```python
from build123d import *

# Parameters (mm, degrees)
SKETCH1_R           = 2.286
BOSS_EXTRUDE1_DEPTH = 7.62
CUT_EXTRUDE1_DEPTH  = 10.16
BOSS_EXTRUDE2_DEPTH = 1.27
SKETCH4_R           = 18.415
CUT_EXTRUDE2_DEPTH  = 2.54
FILLET1_R           = 2.54


with BuildPart() as part:
    # Sketch1 → Boss-Extrude1 (new body)
    with BuildSketch(Plane(origin=(0, 0, 0), x_dir=(1, 0, 0), z_dir=(0, 1, 0))):
        Polygon((5.08, 12.7), (-5.08, 12.7), (-5.08, 10.16), (-15.24, 10.16), (-15.24, 0), (15.24, 0), (15.24, 10.16), (5.08, 10.16), align=None)
        with Locations(Location((-8.89, 5.08, 0), (0, 0, 270))):
            Circle(SKETCH1_R, mode=Mode.SUBTRACT)
        with Locations(Location((8.89, 5.08, 0), (0, 0, 90))):
            Circle(SKETCH1_R, mode=Mode.SUBTRACT)
    extrude(amount=BOSS_EXTRUDE1_DEPTH)

    # Sketch2 → Cut-Extrude1 (cut)
    with BuildSketch(Plane(origin=(5.08, 0, 0), x_dir=(0, 0, -1), z_dir=(1, 0, 0))):
        with BuildLine():
            Line((2.9845, 9.144), (15.6845, 9.144))
            ThreePointArc((15.6845, 9.144), (18.618869601, 5.27151286), (14.097, 3.494049241))
            ThreePointArc((14.097, 3.494049241), (12.5095, 3.940098483), (10.922, 3.494049241))
            ThreePointArc((10.922, 3.494049241), (9.3345, 3.048), (7.747, 3.494049241))
            ThreePointArc((7.747, 3.494049241), (6.1595, 3.940098483), (4.572, 3.494049241))
            ThreePointArc((4.572, 3.494049241), (2.9845, 3.048), (1.397, 3.494049241))
            ThreePointArc((1.397, 3.494049241), (-0.1905, 3.940098483), (-1.778, 3.494049241))
            ThreePointArc((-1.778, 3.494049241), (-2.54101286, 3.161630399), (-3.3655, 3.048))
            Line((-3.3655, 3.048), (-3.3655, 9.144))
            Line((-3.3655, 9.144), (2.9845, 9.144))
        make_face()
    extrude(amount=-CUT_EXTRUDE1_DEPTH, mode=Mode.SUBTRACT)

    # Sketch3 → Boss-Extrude2 (add, symmetric)
    with BuildSketch(Plane(origin=(0, 0, 0), x_dir=(0, 0, -1), z_dir=(1, 0, 0))):
        with BuildLine():
            Line((4.8895, 7.62), (4.8895, 6.096))
            ThreePointArc((4.8895, 6.096), (2.9845, 4.191), (1.0795, 6.096))
            Line((1.0795, 6.096), (1.0795, 7.62))
            Line((1.0795, 7.62), (0, 7.62))
            Line((0, 7.62), (0, 3.934139533))
            ThreePointArc((0, 3.934139533), (0.725327968, 3.799255708), (1.397, 3.494049241))
            ThreePointArc((1.397, 3.494049241), (2.9845, 3.048), (4.572, 3.494049241))
            ThreePointArc((4.572, 3.494049241), (6.1595, 3.940098483), (7.747, 3.494049241))
            ThreePointArc((7.747, 3.494049241), (9.3345, 3.048), (10.922, 3.494049241))
            ThreePointArc((10.922, 3.494049241), (11.777159836, 3.850811359), (12.7, 3.934139533))
            Line((12.7, 3.934139533), (12.7, 7.62))
            Line((12.7, 7.62), (11.2395, 7.62))
            Line((11.2395, 7.62), (11.2395, 6.096))
            ThreePointArc((11.2395, 6.096), (9.3345, 4.191), (7.4295, 6.096))
            Line((7.4295, 6.096), (7.4295, 7.62))
            Line((7.4295, 7.62), (4.8895, 7.62))
        make_face()
    extrude(amount=BOSS_EXTRUDE2_DEPTH, both=True)

    # Sketch4 → Cut-Extrude2 (cut, symmetric)
    with BuildSketch(Plane(origin=(0, 0, 0), x_dir=(0, 0, -1), z_dir=(1, 0, 0))):
        with Locations((21.336, -10.18977017)):
            Circle(SKETCH4_R)
    extrude(amount=CUT_EXTRUDE2_DEPTH, both=True, mode=Mode.SUBTRACT)


with BuildPart() as cut_extrude2_kept_piece:
    # of the separate pieces the step leaves, the one the design keeps (cut_extrude2_pieces_kept)
    add(part.part.solids().sort_by_distance((5.08, 0, -12.7))[0])

    # Fillet1
    fillet1_edges = [cut_extrude2_kept_piece.edges().sort_by_distance(p)[0] for p in [
        (0, 4.301003177, -9.972474456),
    ]]
    fillet(fillet1_edges, radius=FILLET1_R)


solid = cut_extrude2_kept_piece.part
```
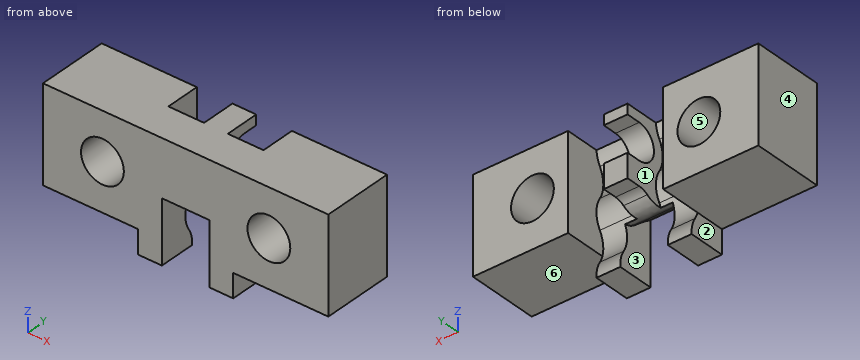
Check sheet for the modelled part. Datum: model origin and axes. Units: mm. Face numbers are marked on the shaded views. A direction names the side the tool comes from. Coordinates: 2 decimals unless noted, no trailing zeros. Order: outer loops, then holes, each group sorted by start corner. A loop starts at its lowest first (then second) coordinate and runs counter-clockwise, first axis right, second up. Notation, with made-up numbers: M 64.5,10.5 L 101.5,10.5 A17 cw 101.5,24.5 Z; hole C 43,62 d5. An arc over 180 degrees is marked long. Write each question's results on one line, items separated by ' | '. Start each with the question number.
1. Cross-section at B-B on y = 5.5. Record the cut outline in (x, z), and give its area (3 significant figures).
2. Material ranges on probe 1 along X at (y, z) = (6.25, -5.08); probe 2 along X at (y, z) = (2, -5.08); probe 3 along X at (y, z) = (4.25, -1.25), recorded low to high.
3. Cross-section at D-D on z = -11.75. Record the cut outline in (x, y).
4. Go/stop test with flat-tipped pins: P1, Ø1.5, axis at x = 7.5, y = 4.5, coming from the -Z side; P2, Ø2, axis at x = 1, y = 2, coming from the -Z side; P3, Ø0.8, axis at y = 2, z = -12, coming from the +X side. Record where each tip stops, or that it passes through.
5. Access from +Z, -Z, +X, -X, +Y, -Y to the whole of each face (thin tool, end or side, straight path). Record for the marked faces 1, 2 and 3.
6. Cross-section at A-A on x = 8.89. Record the cut outline in (y, z).
7. Cross-section at C-C on z = -6.5. Record the cut outline in (x, y).
8. Mould release check, pull along X, two halves, no side actions. Record for the marked faces 4, 5 and 6: +X half, -X half, draft (parallel to the pull), parting line (faces both ways), or undercut.
Checks:
1) outline: M -15.24,-10.16 L -5.08,-10.16 L -5.08,0 L -15.24,0 Z; M -1.27,-7.53 L 1.27,-7.53 L 1.27,-4.79 L -1.27,-4.79 Z; M -1.27,-1.18 L 1.27,-1.18 L 1.27,0 L -1.27,0 Z; M 5.08,-10.16 L 15.24,-10.16 L 15.24,0 L 5.08,0 Z; hole C -8.89,-5.08 d4.57; hole C 8.89,-5.08 d4.57 | area: 184 mm²
2) probe 1: x = -15.24 to -11.18, -6.6 to -5.08, -1.27 to 1.27, 5.08 to 6.6, 11.18 to 15.24 | probe 2: x = -15.24 to -11.18, -6.6 to 6.6, 11.18 to 15.24 | probe 3: x = -15.24 to -5.08, -1.27 to 1.27, 5.08 to 15.24
3) outline: M -5.08,0 L -2.54,0 L -2.54,3.84 L -5.08,3.84 Z; M 2.54,0 L 5.08,0 L 5.08,3.84 L 2.54,3.84 Z
4) P1: stops at z = -10.16 | P2: stops at z = -8.07 | P3: stops at x = 5.08
5) face 1: +Y | face 2: -Z, -X, +Y, -Y | face 3: -Z, -Y
6) outline: M 0,-10.16 L 7.62,-10.16 L 7.62,-7.37 L 0,-7.37 Z; M 0,-2.79 L 7.62,-2.79 L 7.62,0 L 0,0 Z
7) outline: M -15.24,0 L -10.68,0 L -10.68,7.62 L -15.24,7.62 Z; M -7.1,0 L -2.54,0 L -2.54,0.72 L 2.54,0.72 L 2.54,0 L 7.1,0 L 7.1,7.62 L 5.08,7.62 L 5.08,3.92 L 1.27,3.92 L 1.27,7.62 L -1.27,7.62 L -1.27,3.92 L -5.08,3.92 L -5.08,7.62 L -7.1,7.62 Z; M 10.68,0 L 15.24,0 L 15.24,7.62 L 10.68,7.62 Z
8) face 4: -X half | face 5: undercut | face 6: draft
